Source: CAD feature listing. Evaluate the final solid. Frame: model axes, mm. A direction names the side the tool comes from. Round coordinates to 2 decimals unless told otherwise and drop trailing zeros. Write each loop counter-clockwise with the first axis right and the second up, starting at its lowest first coordinate (ties: lowest second). Pieces come first, ordered by that corner, then holes. Notation, with made-up numbers: M -23,16.5 L 15,16.5 A19 cw 15,30.5 Z; hole C 17.5,-0.5 d5. An arc over 180 degrees is marked long. Put each result on its own line as item: value. Start each with the question number.
Autodesk Inventor part; units mm, degrees
ref_plane "YZ Plane" through (0, 0, 0) normal (1, 0, 0) x (0, 1, 0)
ref_plane "XZ Plane" through (0, 0, 0) normal (0, 1, 0) x (-1, 0, 0)
ref_plane "XY Plane" through (0, 0, 0) normal (0, 0, 1) x (1, 0, 0)
sketch "Sketch10" plane through (0, 0, 0) normal (0, 0, 1) x (1, 0, 0)
  circle A0 centre (0, 0) radius 11
  circle A1 centre (0, 0) radius 15
  line L0 (0, 11) -> (0, 35)
  line L1 (0, 35) -> (4.8, 35)
  line L2 (4.8, 35) -> (4.8, 11)
  line L3 (4.8, 11) -> (0, 11)
  line L4 (0, 11) -> (24, 11) construction
  line L5 (4.8, 11) -> (4.8, 35)
  line L6 (4.8, 35) -> (-4.8, 35)
  line L7 (-4.8, 35) -> (-4.8, 11)
  line L8 (-4.8, 11) -> (4.8, 11)
  point P0 (-4.8, 14.2113)
  point P1 (4.8, 14.2113)
  dimension "d75" = 22
  dimension "d76" = 30
  dimension "d77" = 24
  dimension "d78" = 90
  dimension "d79" = 4.8
  dimension "d80" = 9.6
extrude "Extrusion8" add sketch "Sketch10" along normal blind 4.6
fillet "Fillet6" radius 2 5 edges at (4.8, 24.6056, 0) (-4.8, 24.6056, 0) (0, -15, 0) (4.8, 14.2113, 2.3) (-4.8, 14.2113, 2.3)
fillet "Fillet7" radius 2 1 edges at (-11, 0, 0)
properties part number "A1 Holder"
(1) Section query B-B (z = 3.05). Return loops of the section in (x, y).
(2) Ray query, line 1 along X through (y, z) = (0, 3); line 2 along Y through (x, z) = (0, 3.45); line 3 along Z through (x, y) = (3, 22.5). Return the intervals inside material, ascending.
(3) Section query C-C (y = 17). Return loops of the section in (x, z), and give its area (3 significant figures).
(4) Contact query for flat-ended pins moving along their axis: P1, Ø13, axis at x = 0, y = 0, coming from the +Z side; P2, Ø1.3, axis at y = 29.5, z = 3, coming from the +X side; P3, Ø2, axis at y = 25.5, z = 3.5, coming from the -X side. Output: stop coordinate, or through.
(5) Access query for faces 5 (the flat face through (4.8, 25, 3)), 6 (the flat face through (0, 35, 2)), 7 (the cylindrical face through (-4.23, 25.15, 0.6)), 8 (the flat face through (-4.8, 25, 3)), 9 (the cylindrical face through (4.2, 25.15, 0.57)). Directions: +Z, -Z, +X, -X, +Y, -Y. A direction counts if a zero-diameter tool reaches every point of the face in a straight line with its end or side. Return the directions, or none.
(6) Pull-direction query (X, two-part tool) for faces 1 (the cylindrical face through (-5.136, 14.472, 3.318)), 2 (the cylindrical face through (5.118, 14.499, 3.318)), 3 (the flat face through (-7, 10, 4.6)), 4 (the cylindrical face through (-2.38, 10.74, 3.28)); classes: +X half, -X half, draft (parallel to the pull), parting line (faces both ways), or undercut.
Entries:
1. outline: M -6,13.75 A15 ccw long 6,13.75 A2 cw 4.8,15.58 L 4.8,35 L -4.8,35 L -4.8,15.58 A2 cw Z; hole C 0,0 d22
2. line 1: -15 to -11, 11 to 15
2. line 2: -15 to -11, 11 to 35
2. line 3: 0.01 to 4.6
3. outline: M -4.8,2 A2 ccw -2.8,0 L 2.8,0 A2 ccw 4.8,2 L 4.8,4.6 L -4.8,4.6 Z
3. area: 42.4 mm2
4. P1: through
4. P2: x = 4.8
4. P3: x = -4.8
5. face 5: +Z, -Z, +X, +Y
5. face 6: +Z, -Z, +X, -X, +Y
5. face 7: -Z, -X, +Y
5. face 8: +Z, -Z, -X, +Y
5. face 9: -Z, +X, +Y
6. face 1: -X half
6. face 2: +X half
6. face 3: draft
6. face 4: undercut
